Input: part model. Units: mm. Frame: model coordinates. A direction names the side the tool comes from. Coordinates: 2 decimals unless noted, no trailing zeros. Order: outer loops, then holes, each group sorted by start corner. A loop starts at its lowest first (then second) coordinate and runs counter-clockwise, first axis right, second up. Notation, with made-up numbers: (21, -15.5) -> (36, -15.5) arc R19 cw to (36, -9.5) -> close; hole circle Ø8 at (72, 76). An arc over 180 degrees is marked (long way). One line per question, with ' | ' between items.
```python
from build123d import *

# Parameters (mm, degrees)
PAD7367_DEPTH          = 254
POCKET686_DEPTH        = 63.501
LINEARPATTERN003_COUNT = 15
LINEARPATTERN003_PITCH = 14.514286
FILLET569_R            = 6.35
FILLET570_R            = 3.175


with BuildPart() as part:
    # Sketch8382 → Pad7367 (new body)
    with BuildSketch(Plane.YZ):
        Polygon((-38.1, -63.5), (-38.1, 0), (38.1, 0), (38.1, -63.5), (34.925, -63.5), (34.925, -3.175), (-34.925, -3.175), (-34.925, -63.5), align=None)
    extrude(amount=-PAD7367_DEPTH)

    # Sketch8384 → Pocket686 (cut, through all)
    with BuildSketch(Plane.XY):
        with BuildLine():
            ThreePointArc((-28.575, -25.4), (-25.4, -28.575), (-22.225, -25.4))
            Line((-22.225, -25.4), (-22.225, 25.4))
            ThreePointArc((-22.225, 25.4), (-25.4, 28.575), (-28.575, 25.4))
            Line((-28.575, 25.4), (-28.575, -25.4))
        make_face()
    pocket686 = extrude(amount=-POCKET686_DEPTH, mode=Mode.SUBTRACT)

    # LinearPattern003: Pocket686 ×15
    with Locations(*[(-i * LINEARPATTERN003_PITCH, 0, 0) for i in range(1, LINEARPATTERN003_COUNT)]):
        add(pocket686, mode=Mode.SUBTRACT)

    # Fillet569
    fillet569_edges = [part.edges().sort_by_distance(p)[0] for p in [
        (-127, -38.1, 0),
        (-127, 38.1, 0),
    ]]
    fillet(fillet569_edges, radius=FILLET569_R)

    # Fillet570
    fillet570_edges = [part.edges().sort_by_distance(p)[0] for p in [
        (-127, -34.925, -3.175),
        (-127, 34.925, -3.175),
    ]]
    fillet(fillet570_edges, radius=FILLET570_R)


with BuildPart() as part_1:
    # Body6681 placement: moved
    add(part.part.moved(Location((381, 0, 63.5))))


solid = part_1.part
```
1. Pin query (flat end, axial travel): pin 1 Ø1.5 at (x, y) = (278, 22) entering from -Z (3 decimals). Return the tip coordinate at first contact, or that it passes through.
Recorded:
pin 1: stops at z = 60.325
2. Cut plane C-C, the plane y = -15. State how many separate pieces and enclosed holes the cut face has, and give its area (3 significant figures).
Recorded:
separate pieces: 16 | enclosed holes: 0 | area: 504 mm^2
3. Cut plane B-B, the plane x = 355.6. Return loops of the section in (y, z) (3 decimals).
Recorded:
outline: (-38.1, 0) -> (-34.925, 0) -> (-34.925, 57.15) arc R3.175 cw to (-31.75, 60.325) -> (-28.575, 60.325) -> (-28.575, 63.5) -> (-31.75, 63.5) arc R6.35 ccw to (-38.1, 57.15) -> close; (28.575, 60.325) -> (31.75, 60.325) arc R3.175 cw to (34.925, 57.15) -> (34.925, 0) -> (38.1, 0) -> (38.1, 57.15) arc R6.35 ccw to (31.75, 63.5) -> (28.575, 63.5) -> close
4. Cut plane A-A, the plane z = 36. Return loops of the section in (x, y) (3 decimals).
Recorded:
outline: (127, -38.1) -> (381, -38.1) -> (381, -34.925) -> (127, -34.925) -> close; (127, 34.925) -> (381, 34.925) -> (381, 38.1) -> (127, 38.1) -> close
5. Ray query, line 1 (Y direction, x = 235, z = 51.5) (3 decimals); line 2 (Z direction, x = 334.5, y = -10) (3 decimals); line 3 (Z direction, x = 263, y = -32.5). Return the intervals inside material, ascending. Write a range as [from, to].
Recorded:
line 1: y = [-38.1, -34.925], [34.925, 38.1] | line 2: z = [60.325, 63.5] | line 3: z = [60.24, 63.46]
6. Access query for faces 1 (the face through (256, 34.925, 28)), 2 (the face through (256, 38.1, 29)). Directions: +Z, -Z, +X, -X, +Y, -Y. A direction counts if a zero-diameter tool reaches every point of the face in a straight line with its end or side. Return the directions, or none.
Recorded:
face 1: -Z, +X, -X | face 2: +Z, -Z, +X, -X, +Y
7. Cut plane D-D, the plane x = 145.5. Return loops of the section in (y, z) (3 decimals).
Recorded:
outline: (-38.1, 0) -> (-34.925, 0) -> (-34.925, 57.15) arc R3.175 cw to (-31.75, 60.325) -> (31.75, 60.325) arc R3.175 cw to (34.925, 57.15) -> (34.925, 0) -> (38.1, 0) -> (38.1, 57.15) arc R6.35 ccw to (31.75, 63.5) -> (-31.75, 63.5) arc R6.35 ccw to (-38.1, 57.15) -> close
8. Mould query, pull axis Y, two halves, no side actions, for faces 3 (the face through (252.22, 36.19, 61.69)), 4 (the face through (256, -34.925, 29)), 5 (the face through (127, 0, 62)), 6 (the face through (252.22, -36.29, 61.59)). Classes: released by +Y, released by -Y, zero draft, split by the parting line, or undercut.
Recorded:
face 3: released by +Y | face 4: undercut | face 5: zero draft | face 6: released by -Y
